Autodesk Inventor part; units mm, degrees
ref_plane "WorkPlane2" through (0, 0, 0) normal (0, 0, 1) x (1, 0, 0)
ref_plane "Work Plane2" through (0, 0, -2.35) normal (0, 0, 1) x (1, 0, 0)
ref_plane "WorkPlane3" through (0, 0, 7) normal (0, 0, 1) x (1, 0, 0)
ref_plane "WorkPlane2" through (0, 0, 0) normal (0, 0, 1) x (1, 0, 0)
sketch "Sketch1" plane through (0, 0, 0) normal (1, 0, 0) x (0, 1, 0)
  point P0 (0, 0)
ref_plane "Work Plane2" through (0, 0, -2.35) normal (0, 0, 1) x (1, 0, 0)
ref_plane "WorkPlane3" through (0, 0, 7) normal (0, 0, 1) x (1, 0, 0)
sketch "Sketch2" plane through (0, 0, 0) normal (0, 1, 0) x (-1, 0, 0)
  point P0 (0, 0)
sketch "Sketch3" plane through (0, 0, 0) normal (1, 0, 0) x (0, 1, 0)
  line L0 (1.5, -3.35) -> (1.25, -2.85)
  line L1 (1.5, -30.7) -> (1.5, -3.35)
  line L2 (0, -30.7) -> (1.5, -30.7)
  line L3 (0, 0) -> (0, -30.7)
  arc A0 (2.75, -0.7) -> (0, 0) centre (0, -5.7518) ccw
  line L4 (2.75, -0.85) -> (2.75, -0.7)
  line L5 (1.25, -2.35) -> (2.75, -0.85)
  line L6 (1.25, -2.85) -> (1.25, -2.35)
  line L7 (0, -31.6445) -> (0, 31.6445) construction
  line L8 (0, -31.6445) -> (0, 31.6445)
  line L9 (0, -44.3023) -> (0, 44.3023)
  dimension "d2" = 1.5
  dimension "d4" = 1.25
  dimension "d6" = 0.5
  dimension "d8" = 1.65
  dimension "d10" = 135
  dimension "d12" = 2.75
  dimension "d14" = 0
  dimension "d16" = 0.7
  dimension "d18" = 30
  dimension "d22" = 27.35
revolve "Revolution1" add sketch "Sketch3" angle 360 about axis through (0, 0, -31.6445) along (0, 0, 1)
fillet "Fillet1" radius 0.8 1 edges at (0, -1.25, -2.35)
sketch "Sketch4" plane through (0, 0, 0) normal (0, 1, 0) x (-1, 0, 0)
  line L0 (0, 0) -> (-1.7, 0)
  line L1 (0, -1.4167) -> (0, 0)
  line L2 (-1.7, 0) -> (-0.2833, -1.4167)
  line L3 (0, -6.9021) -> (0, 1.1504)
  arc A0 (2.75, -0.7) -> (-2.75, -0.7) centre (0, -5.7518) ccw
  line L4 (0, -1.4167) -> (-0.2833, -1.4167)
  point P0 (0, -1.7)
  dimension "d30" = 45
  dimension "d33" = 3.4
  dimension "d34" = 0.2833
  dimension "d35" = 90
extrude "Extrusion1" cut sketch "Sketch4" along normal mid plane 0.5667
pattern_circular "PolarArray1" count 4 over 360 about axis through (0, 0, -10) along (0, 0, 1) of "Extrusion1"
thread "Thread1"
ref_plane "MSC_PF1" through (0, 0, 0) normal (1, 0, 0) x (0, 1, 0)
ref_plane "MSC_PT1" through (0, 2.75, -0.85) normal (0, 0, -1) x (-1, 0, 0)
equation "\"d2\" = 0.5 * NND"
equation "\"d4\" = 0.5 * msp_mdtds"
equation "\"d6\" = msp_x"
equation "\"d8\" = ParK"
equation "\"d12\" = 0.5 * Dk"
equation "\"d16\" = ParF"
equation "\"d18\" = NLG"
equation "\"d22\" = b"
equation "\"d24\" = r"
equation "\"d33\" = M"
equation "\"d31\" = 0.166667 * M"
equation "\"d39\" = b"
equation "\"PTC\" = 0.5"
equation "\"msp_x\" = PTC"
equation "\"NLG\" = 30"
equation "\"NND\" = 3"
equation "\"ParK\" = 1.65"
equation "\"r\" = 0.8"
equation "\"msp_mdtds\" = NND - PTC"
equation "\"b\" = 27.35"
equation "\"Dk\" = 5.5"
equation "\"ParF\" = 0.7"
equation "\"M\" = 3.4"
equation "\"ParA\" = 1"
equation "\"THREADDIA\" = NND"
equation "\"TEMPLATE\" = 1.2345"
properties part number "ISO 7047 - M3x30 - 4.8 - H" material "Steel"
Could you check a few things on this model? Use its own coordinates, in mm. Round coordinates to 2 decimals unless told otherwise and drop trailing zeros. Loops run counter-clockwise (first coordinate to the right, second up) from the corner with the lowest first, then second, coordinate; pieces in that order, holes last.
Q1. I want a section at A-A (z = -7.5). Write out the boundary of the cut face in (x, y).
Q2. Thinking about a two-plate mould opening in X: for faces 1 (the flat face through (0, -0.9, -0.8)), 2 (the cylindrical face through (-0.07, -1.5, -16.83)), 3 (the flat face through (0, 0, -30.7)), which applies, pulls with the +X half, pulls with the -X half, needs draft (parallel to the pull), parting line crosses it, or undercut?
Q3. For P1, Ø0.6, axis at x = -1, z = -0.5, coming from the -Y side; P2, Ø2, axis at y = 0.5, z = -14, coming from the -X side; P3, Ø2, axis at x = 0, z = -15.5, coming from the -Y side, each with a flat end and sliding along its axis, tell me the tip position at first contact or that it passes through.
Q4. Please list where these lines run through material, in increasing order: L1, parallel to Z at x = 0.2, y = 0.2; L2, parallel to X at y = -0.05, z = -14.5; L3, parallel to Z at x = 1, y = 1.9.
Answer below:
1. outline: circle Ø3 at (0, 0)
2. face 1: undercut
2. face 2: parting line crosses it
2. face 3: needs draft
3. P1: stops at y = -2.64
3. P2: stops at x = -1.5
3. P3: stops at y = -1.5
4. L1: z = -30.7 to -1.42
4. L2: x = -1.5 to 1.5
4. L3: z = -1.45 to -0.42
